from build123d import *

# Parameters (mm, degrees)
ESQUISSE1_R                  = 67.85
ESQUISSE1_R_2                = 50
BOSS_EXTRU_1_DEPTH           = 71.4
ESQUISSE3_R                  = 135.7
ESQUISSE3_R_2                = 50
BOSS_EXTRU_2_DEPTH           = 64.3
ENL_V_MAT_EXTRU_1_DEPTH      = 236.039294587
ENL_V_MAT_EXTRU_1_DEPTH_BACK = 236.039294587
ESQUISSE4_R                  = 14.3
ENL_V_MAT_EXTRU_2_DEPTH      = 236.03929476
ENL_V_MAT_EXTRU_3_DEPTH      = 235.903107858
ENL_V_MAT_EXTRU_3_DEPTH_BACK = 235.903107858
ESQUISSE7_R                  = 7.15


with BuildPart() as part:
    # Esquisse1 → Boss.-Extru.1 (new body)
    with BuildSketch(Plane.XY):
        Circle(ESQUISSE1_R)
        Circle(ESQUISSE1_R_2, mode=Mode.SUBTRACT)
    extrude(amount=-BOSS_EXTRU_1_DEPTH)

    # Esquisse3 → Boss.-Extru.2 (add)
    with BuildSketch(Plane(origin=(0, 0, -71.4), x_dir=(-1, 0, 0), z_dir=(0, 0, -1))):
        Circle(ESQUISSE3_R)
        with Locations(Location((0, 0, 0), (0, 0, 180))):
            Circle(ESQUISSE3_R_2, mode=Mode.SUBTRACT)
    extrude(amount=BOSS_EXTRU_2_DEPTH)

    # Esquisse4 → Enlèv. mat.-Extru.1 (cut, two sides: drawn at the far end of the back side and taken through both)
    with BuildSketch(Plane(origin=(0, 0, 0), x_dir=(0, 0, -1), z_dir=(1, 0, 0)).offset(-ENL_V_MAT_EXTRU_1_DEPTH_BACK)):
        with Locations(Location((71.4, 0, 0), (0, 0, 180))):
            Circle(ESQUISSE4_R)
    extrude(amount=ENL_V_MAT_EXTRU_1_DEPTH + ENL_V_MAT_EXTRU_1_DEPTH_BACK, mode=Mode.SUBTRACT)

    # Esquisse6 → Enlèv. mat.-Extru.2 (cut, through all)
    with BuildSketch(Plane(origin=(0, 0, -135.7), x_dir=(-1, 0, 0), z_dir=(0, 0, -1))):
        with BuildLine():
            Line((-8, 105.7), (8, 105.7))
            Line((8, 105.7), (8, 135.463980452))
            ThreePointArc((8, 135.463980452), (0, 135.7), (-8, 135.463980452))
            Line((-8, 135.463980452), (-8, 105.7))
        make_face()
        with BuildLine():
            Line((8, -105.7), (8, -135.463980452))
            ThreePointArc((8, -135.463980452), (0, -135.7), (-8, -135.463980452))
            Line((-8, -135.463980452), (-8, -105.7))
            Line((-8, -105.7), (8, -105.7))
        make_face()
    extrude(amount=-ENL_V_MAT_EXTRU_2_DEPTH, mode=Mode.SUBTRACT)

    # Esquisse7 → Enlèv. mat.-Extru.3 (cut, two sides: drawn at the far end of the back side and taken through both)
    with BuildSketch(Plane(origin=(0, 0, 0), x_dir=(0, 0, -1), z_dir=(1, 0, 0)).offset(-ENL_V_MAT_EXTRU_3_DEPTH_BACK)):
        with Locations((103.55, 114.063980452)):
            Circle(ESQUISSE7_R)
        with Locations((103.55, -114.063980452)):
            Circle(ESQUISSE7_R)
    extrude(amount=ENL_V_MAT_EXTRU_3_DEPTH + ENL_V_MAT_EXTRU_3_DEPTH_BACK, mode=Mode.SUBTRACT)


solid = part.part
Read the model definition and answer for the solid it produces. Units are mm, in the model's axes. A direction names the side the tool comes from. Round coordinates to 2 decimals unless told otherwise and drop trailing zeros. Loops run counter-clockwise (first coordinate to the right, second up) from the corner with the lowest first, then second, coordinate; pieces in that order, holes last.
Q1. Section C-C on z = -91 is taken. Write down the section's boundary in (x, y), and give its area (3 significant figures).
Q2. Determine the mould class of faces 1 (the face through (2, -74, -71.4)), 2 (the face through (0, 105.7, -104)), 3 (the face through (-82.666, -0.629, -85.686)) for opening direction Z: released by +Z, released by -Z, zero draft, split by the parting line, or undercut.
Q3. Each of these flat-tipped pins is pushed along its axis until it touches: pin 1 (12 mm diameter, centred on y = -76, z = -44.5, fed in from +X); pin 2 (8 mm diameter, centred on x = 3.5, z = -115, fed in from +Y); pin 3 (12 mm diameter, centred on y = 97.5, z = -95, fed in from +X); pin 4 (18.5 mm diameter, centred on y = -114.06, z = -103.55, fed in from +X). Where does it stop, or does it pass through?
Q4. Consider probe 1 along Y at (x, z) = (27, -103); probe 2 along Y at (x, z) = (39.5, -103.55); probe 3 along Y at (x, z) = (-87, -82). Determine where each line is inside the solid, lowest interval first.
Q5. Which of the six approach directions +Z, -Z, +X, -X, +Y, -Y give full straight-line access (tool end or side, diameter ignored) to faces 4 (the face through (2, 76, -71.4)), 5 (the face through (-8, -124, -104)), 6 (the face through (-8, 124, -104))?
Q6. Section D-D on y = -33 is taken. Write down the section's boundary in (x, z).
Q7. Section A-A on y = 0 is taken. Write down the section's boundary in (x, z).
Q8. Section B-B on x = 0 is taken. Write down the section's boundary in (y, z), and give its area (3 significant figures).
Output:
1. outline: (-8, -135.46) - (-8, -105.7) - (8, -105.7) - (8, -135.46) arc R135.7 ccw to (8, 135.46) - (8, 105.7) - (-8, 105.7) - (-8, 135.46) arc R135.7 ccw to start; hole circle Ø100 at (0, 0)
1. area: 49,000 mm2
2. face 1: released by +Z
2. face 2: zero draft
2. face 3: undercut
3. pin 1: passes through
3. pin 2: stops at y = 105.7
3. pin 3: stops at x = 100.21
3. pin 4: stops at x = 86.19
4. probe 1: y = -132.99 to -121.19, -106.94 to -42.08, 42.08 to 106.94, 121.19 to 132.99
4. probe 2: y = -129.82 to -121.21, -106.91 to -30.66, 30.66 to 106.91, 121.21 to 129.82
4. probe 3: y = -104.14 to -9.6, 9.6 to 104.14
5. face 4: +Z, +Y
5. face 5: +Z, -Z, -Y
5. face 6: +Z, -Z, +Y
6. outline: (-131.63, -135.7) - (-37.56, -135.7) - (-37.56, 0) - (-59.28, 0) - (-59.28, -71.4) - (-131.63, -71.4) - close; (37.56, -135.7) - (131.63, -135.7) - (131.63, -71.4) - (59.28, -71.4) - (59.28, 0) - (37.56, 0) - close
7. outline: (-135.7, -135.7) - (-50, -135.7) - (-50, -85.7) - (-135.7, -85.7) - close; (-67.85, -57.1) - (-50, -57.1) - (-50, 0) - (-67.85, 0) - close; (50, -135.7) - (135.7, -135.7) - (135.7, -85.7) - (50, -85.7) - close; (50, -57.1) - (67.85, -57.1) - (67.85, 0) - (50, 0) - close
8. outline: (-105.7, -135.7) - (-50, -135.7) - (-50, 0) - (-67.85, 0) - (-67.85, -71.4) - (-105.7, -71.4) - close; (50, -135.7) - (105.7, -135.7) - (105.7, -71.4) - (67.85, -71.4) - (67.85, 0) - (50, 0) - close
8. area: 9,710 mm2
